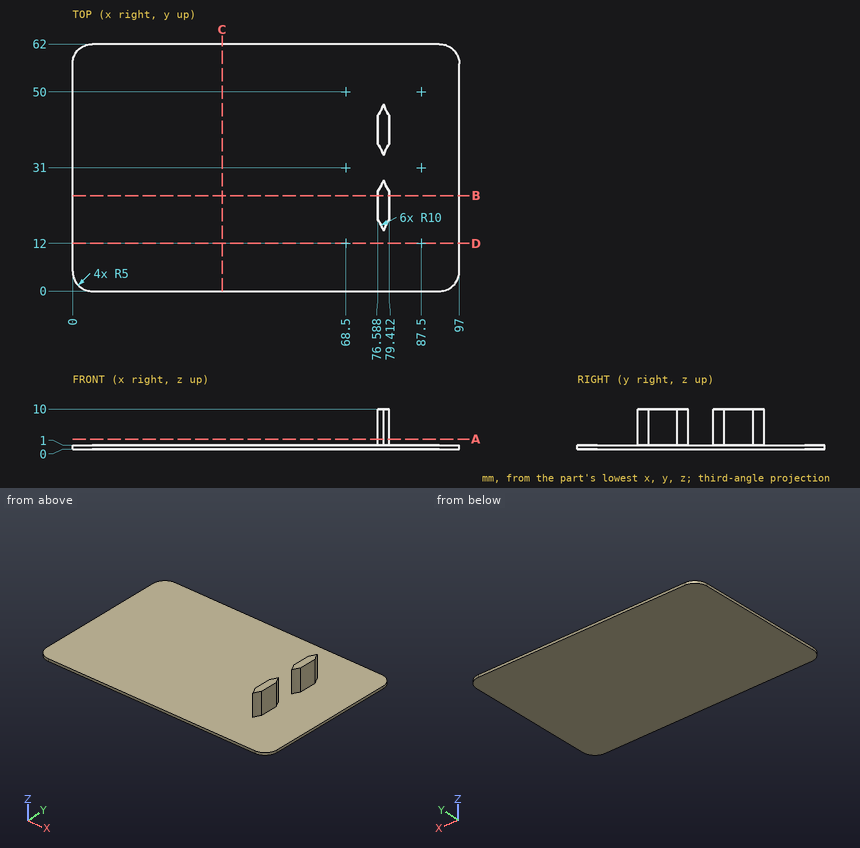
Can you work these out from the drawing? Everything is in mm from the part's minimum corner. Coordinates: 2 decimals unless noted, no trailing zeros. Loops run counter-clockwise (first coordinate to the right, second up) from the corner with the lowest first, then second, coordinate; pieces in that order, holes last.
1. Imagine slicing it at D-D, the plane y = 12. Please give me the cut outline in (x, z).
2. I need wall thicknesses on L1, parallel to Z at x = 32.5, y = 52.5; L2, parallel to X at y = 18, z = 9.5; L3, parallel to X at y = 44.5, z = 9.25. Which ranges of each line are inside material? Lowest first, please.
3. For P1, Ø6, axis at y = 39, z = 7.5, coming from the +X side; P2, Ø4, axis at x = 62.5, z = 4.5, coming from the +Y side (3 decimals); P3, Ø6, axis at y = 55, z = 3.5, coming from the +X side; P4, Ø2, axis at y = 34.5, z = 7.5, coming from the +X side, each with a flat end and sliding along its axis, tell me the tip position at first contact or that it passes through.
4. Imagine slicing it at B-B, the plane y = 24. Please give me the cut outline in (x, z), and give its area (3 significant figures).
5. Imagine slicing it at A-A, the plane z = 2.5. Please give me the cut outline in (x, y), and give its area (3 significant figures).
6. Imagine slicing it at C-C, the plane x = 37.5. Please give me the cut outline in (y, z).
Taken from the geometry:
1. outline: (0, 0) - (97, 0) - (97, 1) - (0, 1) - close
2. L1: z = 0 to 1
2. L2: x = 76.59 to 79.41
2. L3: x = 76.85 to 79.15
3. P1: stops at x = 79.41
3. P2: passes through
3. P3: stops at x = 97
3. P4: stops at x = 78.57
4. outline: (0, 0) - (97, 0) - (97, 1) - (79.41, 1) - (79.41, 10) - (76.59, 10) - (76.59, 1) - (0, 1) - close
4. area: 122 mm2
5. outline: (76.59, 17.88) arc R10 cw to (78, 15.12) arc R10 cw to (79.41, 17.88) - (79.41, 25.12) arc R10 cw to (78, 27.88) arc R10 cw to (76.59, 25.12) - close; (76.59, 36.88) arc R10 cw to (78, 34.12) arc R10 cw to (79.41, 36.88) - (79.41, 44.12) arc R10 cw to (78, 46.88) arc R10 cw to (76.59, 44.12) - close
5. area: 54.5 mm2
6. outline: (0, 0) - (62, 0) - (62, 1) - (0, 1) - close
